Autodesk Inventor part; units mm, degrees
ref_plane "YZ Plane" through (0, 0, 0) normal (1, 0, 0) x (0, 1, 0)
ref_plane "XZ Plane" through (0, 0, 0) normal (0, 1, 0) x (-1, 0, 0)
ref_plane "XY Plane" through (0, 0, 0) normal (0, 0, 1) x (1, 0, 0)
sketch "草圖1" plane through (0, 0, 0) normal (0, 1, 0) x (-1, 0, 0)
  line L0 (0, 0) -> (-70, 0)
  line L1 (-70, 0) -> (-70, -40)
  line L2 (-70, -40) -> (0, -40)
  line L3 (0, -40) -> (0, 0)
  dimension "d0" = 40
  dimension "d1" = 70
extrude "擠出1" add sketch "草圖1" along normal blind 20
sketch "草圖2" plane through (0, 0, 0) normal (0, 0, 1) x (1, 0, 0)
  line L0 (0, 20) -> (70, 20)
  line L1 (0, 20) -> (10, 20)
  line L2 (10, 20) -> (10, 40)
  line L3 (10, 40) -> (0, 40)
  line L4 (0, 40) -> (0, 20)
  point P0 (0, 0)
  dimension "d4" = 10
  dimension "d5" = 20
extrude "擠出2" add sketch "草圖2" against normal up to surface (40 mm away)
sketch "草圖3" plane through (70, 0, -40) normal (0, 0, -1) x (-1, 0, 0)
  line L0 (60, 20) -> (60, 40)
  line L1 (60, 20) -> (40, 20)
  line L2 (40, 20) -> (40, 40)
  line L3 (40, 40) -> (60, 40)
  line L4 (60, 40) -> (60, 20)
  point P0 (70, 0)
  dimension "d8" = 20
  dimension "d9" = 20
extrude "擠出3" add sketch "草圖3" against normal blind 10
sketch "草圖4" plane through (0, 0, 0) normal (0, 0, 1) x (1, 0, 0)
  line L0 (30, 20) -> (10, 20)
  line L1 (30, 20) -> (30, 40)
  line L2 (30, 40) -> (10, 40)
  line L3 (10, 20) -> (10, 40)
  point P0 (0, 0)
extrude "擠出4" add sketch "草圖4" against normal blind 10
chamfer "倒角1" distance 20 angle 45 1 edges at (30, 40, -5)
fillet "圓角1" radius 10 2 edges at (70, 10, 0) (70, 10, -40)
sketch "草圖5" plane through (0, 20, 0) normal (0, 1, 0) x (1, 0, 0)
  circle A0 centre (50, 20) radius 10
  line L0 (30, 0) -> (60, 0)
  line L1 (70, 10) -> (70, 30)
  point P0 (0, 0)
  dimension "d18" = 20
  dimension "d19" = 20
  dimension "d20" = 20
extrude "擠出5" cut sketch "草圖5" against normal through all
properties part number "2"
Source: CAD feature listing. Evaluate the final solid. Frame: model axes, mm. A direction names the side the tool comes from. Give positions to 0.01 mm unless a question says otherwise; leave off trailing zeros. Write each loop counter-clockwise with the first axis right and the second up, starting at its lowest first coordinate (ties: lowest second). Pieces come first, ordered by that corner, then holes. Notation, with made-up numbers: (-9, -9) -> (-1, -9) arc R17 cw to (-1, -1) -> close; hole circle Ø11 at (52, 2). An arc over 180 degrees is marked (long way). Return JSON: item names as keys, results as strings. Group by question number.
1. Section B-B, the plane z = -23. Output: boundary loops of the cut face in (x, y), then the cut area to 3 significant figures.
2. Access query for faces 1 (the face through (30, 30, -35)), 2 (the face through (9, 40, -24)), 3 (the face through (20, 30, -5)), 4 (the face through (66.99, 10.14, -2.85)), 5 (the face through (18, 28, -10)). Directions: +Z, -Z, +X, -X, +Y, -Y. A direction counts if a zero-diameter tool reaches every point of the face in a straight line with its end or side. Return the directions, or none.
3. Section A-A, the plane x = 50. Output: boundary loops of the cut face in (y, z), then the cut area to 3 significant figures.
4. Section C-C, the plane y = 4. Output: boundary loops of the cut face in (x, z).
5. Mould query, pull axis Z, two halves, no side actions, for faces 6 (the face through (67.15, 10.14, -36.99)), 7 (the face through (35, 0, -20)), 8 (the face through (40, 20, -24)), 9 (the face through (10, 30, -20)). Classes: +Z half, -Z half, draft (parallel to the pull), parting line (faces both ways), or undercut.
6. Material intervals for line 1 (Z direction, x = 50, y = 15.25); line 2 (X direction, y = 15.5, z = -20); line 3 (X direction, y = 36.5, z = -14), sorted ascending. Write a range as from..to.
7. Pin query (flat end, axial travel): pin 1 Ø12 at (x, z) = (50, -20) entering from -Y; pin 2 Ø8 at (y, z) = (29.5, -34.5) entering from +X. Return the tip coordinate at first contact, or that it passes through.
Determined:
{
 "1": {"outline": "(0, 0) -> (40.46, 0) -> (40.46, 20) -> (10, 20) -> (10, 40) -> (0, 40) -> close; (59.54, 0) -> (70, 0) -> (70, 20) -> (59.54, 20) -> close", "area": "1,220 mm2"},
 "2": {"face 1": "+Z, -Z, +X, +Y", "face 2": "+Z, -Z, +X, -X, +Y", "face 3": "+Z, +X, +Y", "face 4": "+Z, +X, +Y, -Y", "face 5": "+X, +Y"},
 "3": {"outline": "(0, -40) -> (20, -40) -> (20, -30) -> (0, -30) -> close; (0, -10) -> (20, -10) -> (20, 0) -> (0, 0) -> close", "area": "400 mm2"},
 "4": {"outline": "(0, -40) -> (60, -40) arc R10 ccw to (70, -30) -> (70, -10) arc R10 ccw to (60, 0) -> (0, 0) -> close; hole circle Ø20 at (50, -20)"},
 "5": {"face 6": "-Z half", "face 7": "draft", "face 8": "undercut", "face 9": "undercut"},
 "6": {"line 1": "z = -40..-30, -10..0", "line 2": "x = 0..40, 60..70", "line 3": "x = 0..10"},
 "7": {"pin 1": "passes through", "pin 2": "stops at x = 30"}
}
